Part model, mm, in its own coordinate system. Face numbers are marked on the shaded views. Coordinates: 2 decimals unless noted, no trailing zeros. Write each loop counter-clockwise with the first axis right and the second up, starting at its lowest first coordinate (ties: lowest second). Pieces come first, ordered by that corner, then holes. Notation, with made-up numbers: (70, 46) - (108, 46) arc R19 ccw to (108, 83) - close; hole circle Ø10 at (-1.75, 84). An arc over 180 degrees is marked (long way). Write each question's results on one line, items separated by ' | '.
Autodesk Inventor part; units mm, degrees
ref_plane "Work Plane2" through (-60, 10, 0) normal (0.9396926, 0, -0.3420201) x (0, 1, 0)
ref_plane "XZ Plane" through (0, 0, 0) normal (0, 1, 0) x (-1, 0, 0)
ref_plane "XY Plane" through (0, 0, 0) normal (0, 0, 1) x (1, 0, 0)
sketch "Sketch1" plane through (0, 0, 0) normal (0, 1, 0) x (-1, 0, 0)
  circle A0 centre (0, 0) radius 20
  circle A1 centre (0, 0) radius 22.5
  dimension "d0" = 40
  dimension "d1" = 45
sketch "Sketch2" plane through (0, 0, 0) normal (0, 0, 1) x (1, 0, 0)
  arc A0 (-60, 0) -> (0, 0) centre (-30, 0) ccw
  dimension "d8" = 30
sweep "Sweep2" add profiles "Sketch1" path "Sketch2"
sketch "Sketch3" plane through (-60, 0, 0) normal (0, 1, 0) x (1, 0, 0)
  circle A0 centre (0, 0) radius 20
  circle A1 centre (0, 0) radius 22.5
  circle A2 centre (60, 0) radius 20
  circle A3 centre (60, 0) radius 22.5
extrude "Extrusion1" add sketch "Sketch3" along normal blind 10
ref_plane "Work Plane1" through (0, 0, 0) normal (0.9396926, 0, -0.3420201) x (0, 1, 0)
sketch "Sketch4" plane through (0, 0, 0) normal (0.9396926, 0, -0.3420201) x (0, 1, 0)
  line L0 (10, -22.5) -> (10, 22.5)
  line L1 (0, 22.5) -> (0, -22.5)
  point P0 (0, 0)
  point P1 (5, 0)
  dimension "d14" = 5
  dimension "d15" = 22.5
  dimension "d16" = 22.5
hole "Hole1" at (0, 5, 0) direction (-0.9396926, 0, 0.3420201) diameter 4.5 end up to surface
sketch "Sketch5" plane through (-60, 10, 0) normal (0, 1, 0) x (1, 0, 0)
  point P0 (60, 0)
  point P1 (0, 0)
  point P2 (0, 0)
ref_plane "Work Plane2" through (-60, 10, 0) normal (0.9396926, 0, -0.3420201) x (0, 1, 0)
sketch "Sketch6" plane through (-60, 10, 0) normal (0.9396926, 0, -0.3420201) x (0, 1, 0)
  line L0 (0, -22.5) -> (0, 22.5)
  line L1 (-10, -22.5) -> (-10, 22.5)
  line L2 (-10, -22.5) -> (0, -22.5)
  line L3 (-10, 22.5) -> (0, 22.5)
  point P0 (-10, 20.5212)
  point P1 (-5, 0)
  dimension "d24" = 5
  dimension "d25" = 22.5
  dimension "d26" = 22.5
hole "Hole2" at (-60, 5, 0) direction (0.9396926, 0, -0.3420201) diameter 4.5 end up to surface
properties part number "Pancake_Flexi Pipe" material "PMMA Plastic"
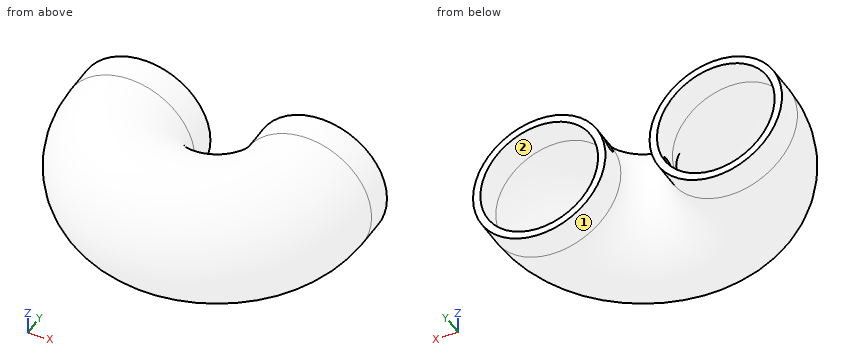
(1) Saw through at B-B on z = -12.5. Write the cut outline in (x, y), then the cut area to 3 significant figures.
Return value:
outline: (-78.71, 0) arc R48.71 ccw to (18.71, 0) - (18.71, 10) - (15.61, 10) - (15.61, 0) arc R45.61 cw to (-75.61, 0) - (-75.61, 10) - (-78.71, 10) - close; (-44.39, 0) arc R14.39 ccw to (-15.61, 0) - (-15.61, 10) - (-18.71, 10) - (-18.71, 0) arc R11.29 cw to (-41.29, 0) - (-41.29, 10) - (-44.39, 10) - close | area: 707 mm^2
(2) Wall check: line 1 (X direction, y = 4, z = 0); line 2 (Z direction, x = -60, y = 2); line 3 (X direction, y = 6, z = 12.5). Give the ranges that are in metal, low to high. Write a range as from..to.
Return value:
line 1: x = -82.5..-80, -40..-37.5, -22.5..-20, 20..22.5 | line 2: z = -22.5..-20, 20..22.5 | line 3: x = -78.71..-75.61, -44.39..-41.29, -18.71..-15.61, 15.61..18.71
(3) Flat gauge pins, fed straight in: P1, Ø12, axis at x = -53.5, y = -6, coming from the +Z side; P2, Ø6, axis at x = -44.5, z = 12.5, coming from the -Y side; P3, Ø5, axis at x = -36.5, y = -37, coming from the +Z side. Where does each tip first touch, or does it go through?
Return value:
P1: stops at z = 22.5 | P2: stops at y = -48.49 | P3: stops at z = 21.92
(4) Saw through at C-C on y = -4. Count the separate pieces of the cut face and the enclosed holes in it, then the cut area to 3 significant figures.
Return value:
separate pieces: 2 | enclosed holes: 2 | area: 687 mm^2
(5) Two-plate mould, pull along Z, no slides. Class the marked faces 1 and 2: released by +Z, released by -Z, zero draft, split by the parting line, or undercut.
Return value:
face 1: split by the parting line | face 2: undercut
(6) Saw through at A-A on z = 0. Write the cut outline in (x, y), then the cut area to 3 significant figures.
Return value:
outline: (-82.5, 0) arc R52.5 ccw to (22.5, 0) - (22.5, 10) - (20, 10) - (20, 0) arc R50 cw to (-80, 0) - (-80, 10) - (-82.5, 10) - close; (-40, 0) arc R10 ccw to (-20, 0) - (-20, 10) - (-22.5, 10) - (-22.5, 0) arc R7.5 cw to (-37.5, 0) - (-37.5, 10) - (-40, 10) - close | area: 571 mm^2
